Source: CAD feature listing. Evaluate the final solid. Frame: model axes, mm. Face numbers are marked on the shaded views. A direction names the side the tool comes from. Give positions to 0.01 mm unless a question says otherwise; leave off trailing zeros. Write each loop counter-clockwise with the first axis right and the second up, starting at its lowest first coordinate (ties: lowest second). Pieces come first, ordered by that corner, then holes. Notation, with made-up numbers: (-21, -2) - (38, -2) arc R18 ccw to (38, 12) - close; hole circle Ø8 at (-23, -23). An arc over 180 degrees is marked (long way). One line per question, with ' | ' between items. Start each with the question number.
(1) Access query for the marked faces 4, 5, 6 and 7. Directions: +Z, -Z, +X, -X, +Y, -Y. A direction counts if a zero-diameter tool reaches every point of the face in a straight line with its end or side. Return the directions, or none.
(2) Section A-A, the plane x = 213.75. State how many separate pieces and enclosed holes the cut face has, plus the area to 3 significant figures.
(3) Pin query (flat end, axial travel): pin 1 (3 mm diameter, centred on y = -25.02, z = 19.33, fed in from +X); pin 2 (10 mm diameter, centred on x = 222, z = 28, fed in from +Y); pin 3 (1.5 mm diameter, centred on x = 209.5, z = -9.5, fed in from +Y); pin 4 (1.3 mm diameter, centred on x = 219, z = -44, fed in from -Y). Return the tip coordinate at first contact, or that it passes through.
(4) Section B-B, the plane z = 38. Return loops of the section in (x, y), plus the area to 3 significant figures.
(5) Draft query along Z for the marked faces 1, 2 and 3. Return one class per face: +Z half, -Z half, draft (parallel to the pull), parting line (faces both ways), or undercut.
(6) Ray query, line 1 (Z direction, x = 217.25, y = 27.5); line 2 (Z direction, x = 212.25, y = -37); line 3 (Y direction, x = 222.25, z = 18). Return the intervals inside material, ascending. Write a range as [from, to].
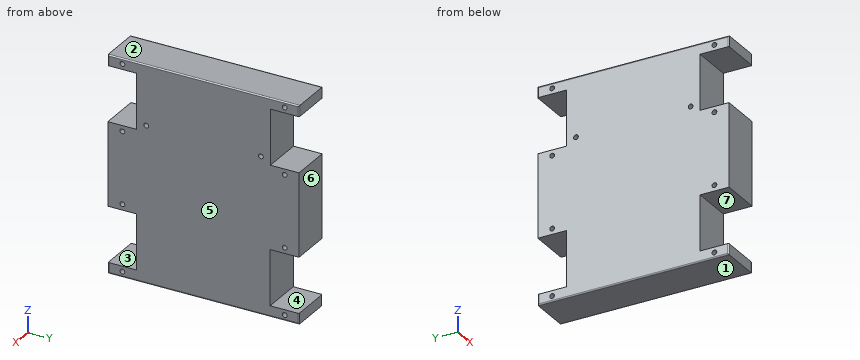
```python
from build123d import *

# Parameters (mm, degrees)
SKETCH2_R           = 25.4
BOSS_EXTRUDE2_DEPTH = 431.8
SCALE1_SCALE        = 0.03937
FILLET2_R           = 0.5


with BuildPart() as part:
    # Sketch2 → Boss-Extrude2 (new body)
    with BuildSketch(Plane(origin=(0, 0, 0), x_dir=(0, 0, -1), z_dir=(1, 0, 0))):
        Polygon((1029.419088994, -710.098177988), (1029.419088994, -1014.561822012), (1143.719088994, -1014.561822012), (1143.719088994, 1014.561822012), (1029.419088994, 1014.561822012), (1029.419088994, 707.221822012), (441.240911006, 707.221822012), (441.240911006, 1014.561822012), (-441.240911006, 1014.561822012), (-441.240911006, 710.098177988), (-1027.980911006, 710.098177988), (-1027.980911006, 1017.438177988), (-1142.280911006, 1017.438177988), (-1142.280911006, -1017.438177988), (-1027.980911006, -1017.438177988), (-1027.980911006, -710.098177988), (-441.240911006, -710.098177988), (-441.240911006, -1017.438177988), (0, -1017.438177988), (442.679088994, -1017.438177988), (442.679088994, -710.098177988), align=None)
        with Locations((1085.85, 862.33)):
            Circle(SKETCH2_R, mode=Mode.SUBTRACT)
        with Locations((381.2428494, 862.33)):
            Circle(SKETCH2_R, mode=Mode.SUBTRACT)
        with Locations((-381.2428494, 862.33)):
            Circle(SKETCH2_R, mode=Mode.SUBTRACT)
        with Locations((-1085.85, 862.33)):
            Circle(SKETCH2_R, mode=Mode.SUBTRACT)
        with Locations((-1085.85, -862.33)):
            Circle(SKETCH2_R, mode=Mode.SUBTRACT)
        with Locations((-381.2428494, -862.33)):
            Circle(SKETCH2_R, mode=Mode.SUBTRACT)
        with Locations((-508, -609.6)):
            Circle(SKETCH2_R, mode=Mode.SUBTRACT)
        with Locations((381.2428494, -862.33)):
            Circle(SKETCH2_R, mode=Mode.SUBTRACT)
        with Locations((1085.85, -862.33)):
            Circle(SKETCH2_R, mode=Mode.SUBTRACT)
        with Locations((-508, 609.6)):
            Circle(SKETCH2_R, mode=Mode.SUBTRACT)
    extrude(amount=BOSS_EXTRUDE2_DEPTH)


with BuildPart() as part_1:
    # Scale1: scaled about (215.9, -1.065263606, -0.699579786)
    add(part.part.scale(SCALE1_SCALE).moved(Location((207.400017, -1.023324178, -0.67203733))))

    # Fillet2
    fillet2_edges = [part_1.edges().sort_by_distance(p)[0] for p in [
        (224.399983, 39.03321689, 42.049566636),
        (224.399983, -1.023324178, 44.299562136),
        (224.399983, -41.079865245, 42.049566636),
        (207.400017, -41.079865245, 42.049566636),
        (207.400017, -1.023324178, 44.299562136),
        (207.400017, 39.03321689, 42.049566636),
        (207.400017, 38.919974755, -43.450262364),
        (207.400017, -1.023324178, -45.700257864),
        (207.400017, -40.96662311, -43.450262364),
        (224.399983, -40.96662311, -43.450262364),
        (224.399983, -1.023324178, -45.700257864),
        (224.399983, 38.919974755, -43.450262364),
    ]]
    fillet(fillet2_edges, radius=FILLET2_R)


solid = part_1.part
```
Check sheet entries:
1) face 4: +X, -X, +Y | face 5: +Z, -Z, +X, +Y, -Y | face 6: -Z, +X, -X, +Y | face 7: +X, -X, -Y
2) separate pieces: 1 | enclosed holes: 10 | area: 6,050 mm²
3) pin 1: x = 224.4 | pin 2: y = 26.93 | pin 3: y = 38.92 | pin 4: y = -40.97
4) outline: (207.4, -28.98) - (224.4, -28.98) - (224.4, 26.93) - (207.4, 26.93) - close | area: 951 mm²
5) face 1: -Z half | face 2: +Z half | face 3: undercut
6) line 1: [-45.7, -41.2], [-18.04, 16.7], [39.8, 44.3] | line 2: [-45.7, -41.2], [-18.1, 16.7], [39.8, 44.3] | line 3: [-28.98, 26.93]
